Autodesk Inventor part; units mm, degrees
ref_plane "YZ Plane" through (0, 0, 0) normal (1, 0, 0) x (0, 1, 0)
ref_plane "XZ Plane" through (0, 0, 0) normal (0, 1, 0) x (-1, 0, 0)
ref_plane "XY Plane" through (0, 0, 0) normal (0, 0, 1) x (1, 0, 0)
sketch "Sketch1" plane through (0, 0, 0) normal (0, 1, 0) x (-1, 0, 0)
  circle A0 centre (0, 0) radius 20
  dimension "d0" = 40
extrude "Extrusion1" add sketch "Sketch1" along normal blind 17
sketch "Sketch2" plane through (0, 17, 0) normal (0, 1, 0) x (1, 0, 0)
  circle A0 centre (-10, 0) radius 1.5
  circle A1 centre (10, 0) radius 1.5
  circle A2 centre (0, 10) radius 1.5
  circle A3 centre (0, -10) radius 1.5
  circle A4 centre (0, 0) radius 4.2
  circle A5 centre (0, 0) radius 5.7
  line L0 (-10, 3.1754) -> (-7.25, 1.5877)
  line L1 (-7.25, 1.5877) -> (-7.25, -1.5877)
  line L2 (-7.25, -1.5877) -> (-10, -3.1754)
  line L3 (-10, -3.1754) -> (-12.75, -1.5877)
  line L4 (-12.75, -1.5877) -> (-12.75, 1.5877)
  line L5 (-12.75, 1.5877) -> (-10, 3.1754)
  line L6 (10, 3.1754) -> (7.25, 1.5877)
  line L7 (7.25, 1.5877) -> (7.25, -1.5877)
  line L8 (7.25, -1.5877) -> (10, -3.1754)
  line L9 (10, -3.1754) -> (12.75, -1.5877)
  line L10 (12.75, -1.5877) -> (12.75, 1.5877)
  line L11 (12.75, 1.5877) -> (10, 3.1754)
  line L12 (1.5877, 12.75) -> (3.1754, 10)
  line L13 (-1.5877, 12.75) -> (1.5877, 12.75)
  line L14 (-3.1754, 10) -> (-1.5877, 12.75)
  line L15 (-1.5877, 7.25) -> (-3.1754, 10)
  line L16 (1.5877, 7.25) -> (-1.5877, 7.25)
  line L17 (3.1754, 10) -> (1.5877, 7.25)
  line L18 (3.1754, -10) -> (1.5877, -7.25)
  line L19 (1.5877, -12.75) -> (3.1754, -10)
  line L20 (-1.5877, -12.75) -> (1.5877, -12.75)
  line L21 (-3.1754, -10) -> (-1.5877, -12.75)
  line L22 (-1.5877, -7.25) -> (-3.1754, -10)
  line L23 (1.5877, -7.25) -> (-1.5877, -7.25)
  dimension "d6" = 3
  dimension "d13" = 8.4
  dimension "d16" = 1.5
sketch "Sketch3" plane through (0, 0, 0) normal (0, -1, 0) x (1, 0, 0)
  circle A0 centre (0, 0) radius 3.5
  dimension "d8" = 7
extrude "Extrusion2" cut sketch "Sketch3" against normal blind 5
extrude "Extrusion4" cut sketch "Sketch2" against normal through all contours A0 | A1 | A2 | A3
extrude "Extrusion5" add sketch "Sketch2" along normal blind 19.75 contours A5
extrude "Extrusion6" add sketch "Sketch2" along normal blind 35.25 contours A4
extrude "Extrusion7" cut sketch "Sketch2" against normal blind 2.4 contours A0 | L0 L1 L2 L3 L4 L5 | L11 L10 L9 L8 L7 L6 | L12 L17 L16 L15 L14 L13 | L19 L20 L21 L22 L23 L18
properties part number "Encoder_coupler_3DPrint"
Design review of the part built by this model. Coordinates are the model's own, in mm. A direction names the side the tool comes from. Coordinates: 2 decimals unless noted, no trailing zeros. Loops run counter-clockwise (first coordinate to the right, second up) from the corner with the lowest first, then second, coordinate; pieces in that order, holes last. Notation, with made-up numbers: M 7,-34.5 L 55,-34.5 A18 cw 55,-23.5 Z; hole C 48,29 d5. An arc over 180 degrees is marked long. One line per question, with ' | ' between items.
(1) We need section C-C (y = 42). Give the boundary of the cut face in (x, z).
Filled in:
outline: C 0,0 d8.4
(2) Machinability: for faces 4 (the face through (2.39, 15.82, 8.64)), 5 (the face through (8.5, 7.4, -0.07)), which of the approach directions +Z, -Z, +X, -X, +Y, -Y give a long, thin tool a straight path to every point of the face, cutting with its end or side? Answer none if there is none.
Filled in:
face 4: +Y | face 5: +Y, -Y
(3) We need section D-D (z = 16.5). Give the boundary of the cut face in (x, y).
Filled in:
outline: M -11.3,0 L 11.3,0 L 11.3,17 L -11.3,17 Z
(4) We need section A-A (x = 0). Count the separate pieces of the cut face and the enclosed holes in it, and give its area (3 significant figures).
Filled in:
separate pieces: 3 | enclosed holes: 0 | area: 886 mm^2
(5) Wall thickness on probe 1 along Z at (x, y) = (0, 1); probe 2 along Z at (x, y) = (0, 9); probe 3 along Y at (x, z) = (-3, -12): over which ranges is each line inside the solid? List them lowest first.
Filled in:
probe 1: z = -20 to -11.5, -8.5 to -3.5, 3.5 to 8.5, 11.5 to 20 | probe 2: z = -20 to -11.5, -8.5 to 8.5, 11.5 to 20 | probe 3: y = 0 to 17
(6) Draft analysis for pull direction X (two halves, no side actions). For faces 1 (the face through (-2, 36.75, 4)), 2 (the face through (4.006, 44.392, 1.262)), 3 (the face through (1.4, 14.6, -11.3)), state which applies: released by +X, released by -X, zero draft, split by the parting line, or undercut.
Filled in:
face 1: zero draft | face 2: split by the parting line | face 3: undercut
(7) For pin 1 Ø1 at (y, z) = (19.5, -1.5) entering from -X; pin 2 Ø5 at (x, y) = (1.5, 43) entering from +Z; pin 3 Ø1.5 at (y, z) = (18, -8) entering from +X; pin 4 Ø3 at (x, z) = (1.5, 9.5) entering from +Y, all flat-tipped, find the tip position at first contact; note any pin that passes through.
Filled in:
pin 1: stops at x = -5.61 | pin 2: stops at z = 4.2 | pin 3: passes through | pin 4: stops at y = 17
(8) We need section B-B (y = 7). Give the boundary of the cut face in (x, z).
Filled in:
outline: C 0,0 d40; hole C -10,0 d3; hole C 0,-10 d3; hole C 0,10 d3; hole C 10,0 d3
